For this review, use the dimensioned drawing (mm, ordinates from the lowest corner) and the shaded views. A direction names the side the tool comes from. Coordinates: 2 decimals unless noted, no trailing zeros. Loops run counter-clockwise (first coordinate to the right, second up) from the corner with the lowest first, then second, coordinate; pieces in that order, holes last.
1. To check wall thickness, follow probe 1 along X at (y, z) = (1.5, 38); probe 2 along Z at (x, y) = (8, 3.5); probe 3 along X at (y, z) = (3.5, 17). State the ranges of each line that lie inside material, in increasing order.
2. Take a section at A-A, the plane x = 31. State the section outline as (y, z) points.
3. Take a section at B-B, the plane z = 27. State the section outline as (x, y) points, then the cut area to 3 significant figures.
4. Clearance check with flat-ended pins moving along their axes: P1, Ø10, axis at x = 29.5, z = 9.5, coming from the +Y side; P2, Ø1.5, axis at y = 5, z = 14.5, coming from the -X side; P3, Ø2.5, axis at x = 4.5, y = 5.5, coming from the -Z side; P4, Ø2.5, axis at x = 4.5, y = 4.5, coming from the +Z side. State where each tip first meets the part, or that it passes through.
5. Take a section at C-C, the plane y = 4. State the section outline as (x, z) points, then the cut area to 3 significant figures.
6. Machinability: for the marked faces 1 and 2, which of the approach directions +Z, -Z, +X, -X, +Y, -Y give a long, thin tool a straight path to every point of the face, cutting with its end or side? Answer none if there is none.
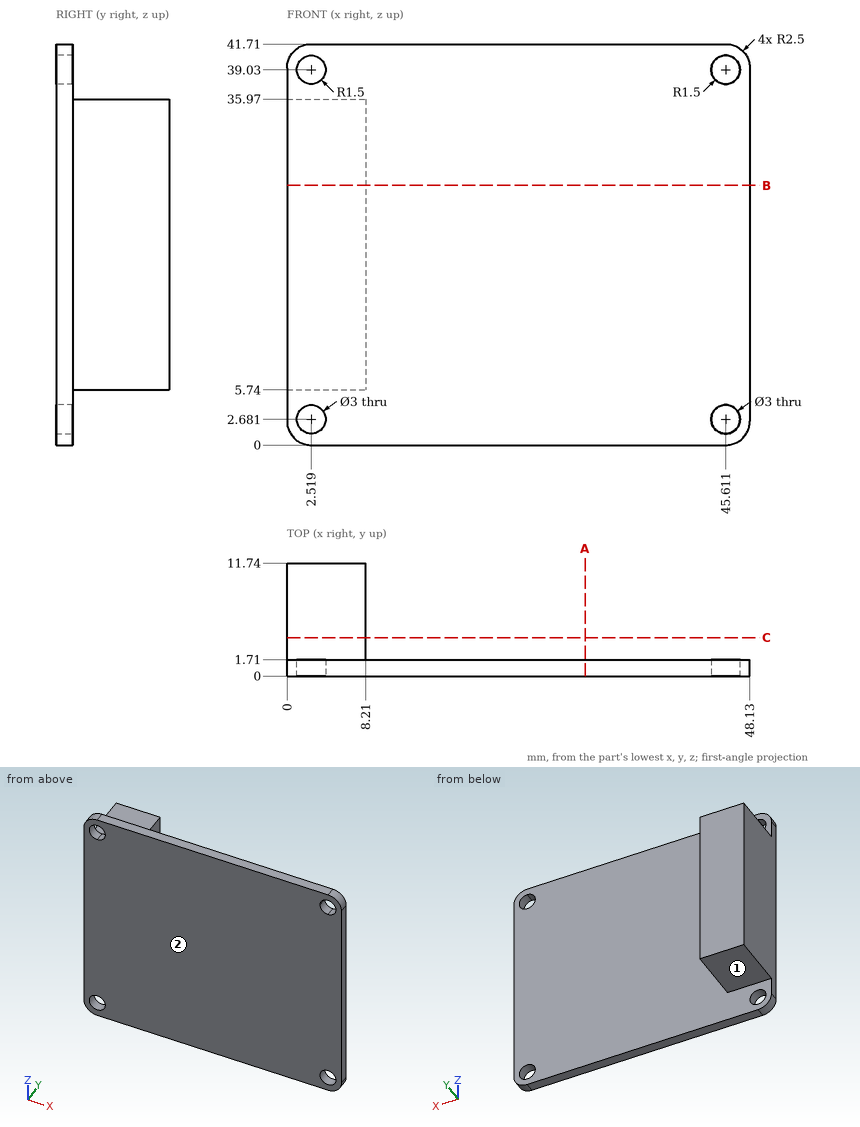
Results list:
1. probe 1: x = 0 to 1.43, 3.61 to 44.52, 46.7 to 48.13
1. probe 2: z = 5.74 to 35.97
1. probe 3: x = 0 to 8.21
2. outline: (0, 0) - (1.71, 0) - (1.71, 41.71) - (0, 41.71) - close
3. outline: (0, 0) - (48.13, 0) - (48.13, 1.71) - (8.21, 1.71) - (8.21, 11.74) - (0, 11.74) - close
3. area: 165 mm2
4. P1: stops at y = 1.71
4. P2: stops at x = 0
4. P3: stops at z = 5.74
4. P4: stops at z = 35.97
5. outline: (0, 5.74) - (8.21, 5.74) - (8.21, 35.97) - (0, 35.97) - close
5. area: 248 mm2
6. face 1: -Z, +X, -X, +Y
6. face 2: +Z, -Z, +X, -X, -Y
